Here's the drawing with two shaded views (mm, measured from the low corner). I have some questions. Round coordinates to 2 decimals unless told otherwise and drop trailing zeros. Loops run counter-clockwise (first coordinate to the right, second up) from the corner with the lowest first, then second, coordinate; pieces in that order, holes last. Notation, with made-up numbers: (32.25, 48.25) - (82.25, 48.25) arc R20 ccw to (82.25, 66.25) - close; hole circle Ø1 at (44.25, -0.75). An arc over 180 degrees is marked (long way). Use one line per item in the form item = value.
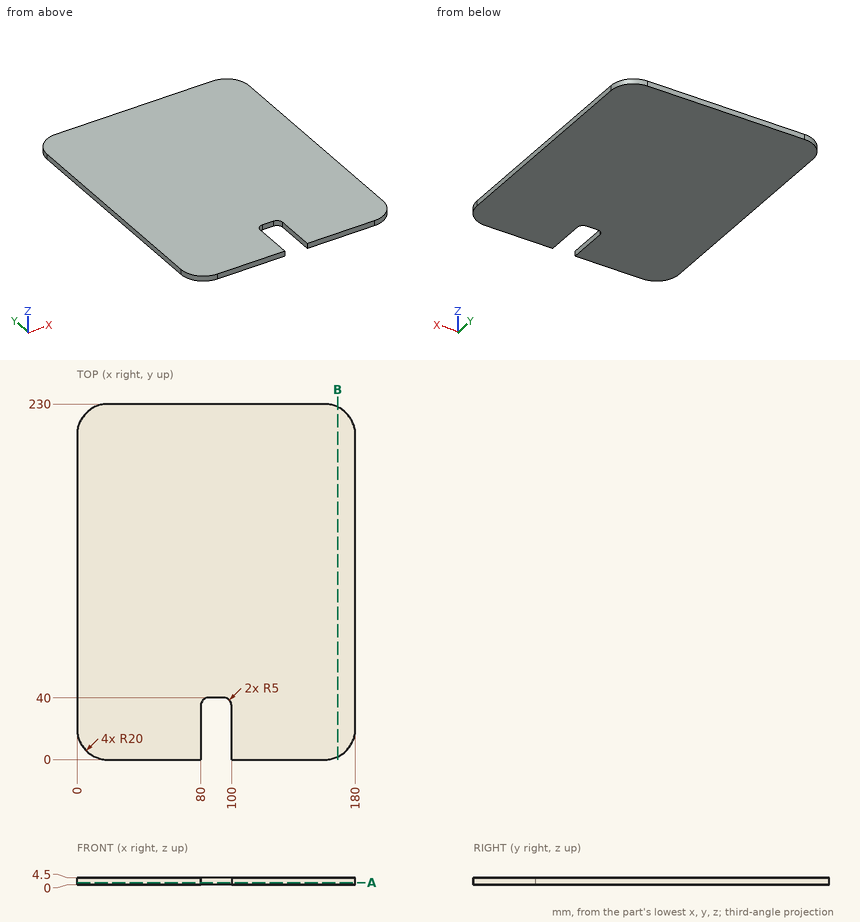
1. For P1, Ø2, axis at y = 16.5, z = 2.5, coming from the +X side, with a flat end and sliding along its axis, tell me the tip position at first contact or that it passes through.
Solution:
P1 = 179.84
2. Please list where these lines run through material, in increasing order: line 1 along X through (y, z) = (212.5, 1.55); line 2 along Y through (x, z) = (163, 3.45); line 3 along Y through (x, z) = (162, 3.95).
Solution:
line_1 = 0.16 to 179.84
line_2 = 0.23 to 229.77
line_3 = 0.1 to 229.9
3. If we section it at B-B, the plane x = 168.5: Write out the boundary of the cut face in (y, z).
Solution:
outline = (1.9, 0) - (228.1, 0) - (228.1, 4.5) - (1.9, 4.5) - close
4. If we section it at A-A, the plane z = 1.3: Write out the boundary of the cut face in (x, y), plus the area to 3 significant figures.
Solution:
outline = (0, 20) arc R20 ccw to (20, 0) - (80, 0) - (80, 35) arc R5 cw to (85, 40) - (95, 40) arc R5 cw to (100, 35) - (100, 0) - (160, 0) arc R20 ccw to (180, 20) - (180, 210) arc R20 ccw to (160, 230) - (20, 230) arc R20 ccw to (0, 210) - close
area = 40,300 mm^2
